Verification items for the finished model (mm, model axes). A direction names the side the tool comes from. Coordinates: 2 decimals unless noted, no trailing zeros. Write each loop counter-clockwise with the first axis right and the second up, starting at its lowest first coordinate (ties: lowest second). Pieces come first, ordered by that corner, then holes. Notation, with made-up numbers: (60.5, -5) -> (80.5, -5) arc R21 ccw to (80.5, 24) -> close; hole circle Ø2 at (-11.5, 78.5). An arc over 180 degrees is marked (long way). Use a Markdown table: item, result. Add a question column.
from build123d import *

# Parameters (mm, degrees)
EXTRUSION1_DEPTH        = 5.25
CONG_1_R                = 2
ENL_V_MAT_EXTRU_1_DEPTH = 2.5


with BuildPart() as part:
    # Esquisse1 → Extrusion1 (new body, symmetric)
    with BuildSketch(Plane.XY):
        with BuildLine():
            Line((4.5, 8), (-4.5, 8))
            Line((-4.5, 8), (-9.009706909, 21.487495824))
            ThreePointArc((-9.009706909, 21.487495824), (0, 34), (9.009706909, 21.487495824))
            Line((9.009706909, 21.487495824), (4.5, 8))
        make_face()
    extrude(amount=EXTRUSION1_DEPTH, both=True)

    # Congé1
    cong_1_edges = [part.edges().sort_by_distance(p)[0] for p in [
        (6.754853455, 14.743747912, 5.25),
        (0, 34, 5.25),
        (-6.754853455, 14.743747912, 5.25),
        (0, 34, -5.25),
        (6.754853455, 14.743747912, -5.25),
        (-6.754853455, 14.743747912, -5.25),
    ]]
    fillet(cong_1_edges, radius=CONG_1_R)

    # Esquisse3 → Révolution2 (revolve)
    with BuildSketch(Plane.XY, mode=Mode.PRIVATE) as r_volution2_sk:
        Polygon((-13.067694578, 46.211312018), (-9.438866144, 31.656876124), (-7.983422555, 32.019758967), (-6.345144878, 25.448986095), (-9.498605988, 24.662739935), (-14.037990304, 45.969390122), align=None)
    r_volution2 = revolve(r_volution2_sk.sketch.rotate(Axis((0, 0, 0), (-0.241921896, 0.970295726, 0)), 180), axis=Axis((0, 0, 0), (-0.241921896, 0.970295726, 0)))  # turned: the seam where the file's is

    # Symétrie1: Révolution2 across plane
    add(r_volution2.mirror(Plane(origin=(0, 0, 0), x_dir=(0, 0, 1), z_dir=(1, 0, 0))))

    # Esquisse5 → Enlèv. mat.-Extru.1 (cut, symmetric)
    with BuildSketch(Plane(origin=(0, 0, 0), x_dir=(0, 0, -1), z_dir=(1, 0, 0))):
        with BuildLine():
            Line((-3.25, 8), (3.25, 8))
            Line((3.25, 8), (3.25, 10))
            Line((3.25, 10), (2.291287847, 10))
            ThreePointArc((2.291287847, 10), (0, 13.5), (-2.291287847, 10))
            Line((-2.291287847, 10), (-3.25, 10))
            Line((-3.25, 10), (-3.25, 8))
        make_face()
    extrude(amount=ENL_V_MAT_EXTRU_1_DEPTH, both=True, mode=Mode.SUBTRACT)


solid = part.part
1) Cross-section at A-A on x = 0. Record the boundary of the cut face in (y, z), then the cut area to 3 significant figures.
2) Thickness scan on L1, parallel to Z at x = 1, y = 11; L2, parallel to X at y = 23.5, z = -3; L3, parallel to X at y = 36.5, z = 2. Record the ranges inside material, lowest first.
3) Cross-section at B-B on z = 4. Record the boundary of the cut face in (x, y).
4) Gauge pin test, flat ends, axial feed: pin 1 (1.1 mm diameter, centred on x = 0, z = -3, fed in from -Y); pin 2 (5 mm diameter, centred on y = 39, z = 3.5, fed in from -X); pin 3 (3 mm diameter, centred on y = 35, z = -3.5, fed in from -X); pin 4 (6 mm diameter, centred on x = 0.5, y = 39.5, fed in from +Z). Record the tip position at first contact, or that the pin passes through.
5) Cross-section at C-C on y = 37.5. Give the number of separate pieces and of enclosed holes in the cut face, then the cut area to 3 significant figures.
6) Release check for a two-part mould opening along Y. For faces 1 (the face through (8.004, 32.015, -0.021)), 2 (the face through (-10.03, 46.97, 0.52)), 3 (the face through (-3, 8, 0)) record: released by +Y, released by -Y, zero draft, split by the parting line, or undercut.
7) Set-up check for faces 4 (the face through (0, 10, 3)), 5 (the face through (0, 13.5, -0.1)), 6 (the face through (-6.11, 14.72, 4.68)): record each of +Z, -Z, +X, -X, +Y, -Y from which the full face is reachable in a straight line by a thin tool's end or side.
Returned:
| question | item | result |
|---|---|---|
| 1 | outline | (8, -5.25) -> (32, -5.25) arc R2 ccw to (34, -3.25) -> (34, 3.25) arc R2 ccw to (32, 5.25) -> (8, 5.25) -> (8, 3.25) -> (10, 3.25) -> (10, 2.29) arc R2.5 cw (long way) to (10, -2.29) -> (10, -3.25) -> (8, -3.25) -> close |
| 1 | area | 244 mm² |
| 2 | L1 | z = -5.25 to -2.5, 2.5 to 5.25 |
| 2 | L2 | x = -9.45 to 9.45 |
| 2 | L3 | x = -11.18 to -6.97, 6.97 to 11.18 |
| 3 | outline | (-8.87, 21.53) -> (-4.35, 8) -> (4.35, 8) -> (8.87, 21.53) arc R9.35 ccw (long way) to start |
| 4 | pin 1 | stops at y = 8 |
| 4 | pin 2 | stops at x = -12.48 |
| 4 | pin 3 | stops at x = -10.91 |
| 4 | pin 4 | passes through |
| 5 | separate pieces | 2 |
| 5 | enclosed holes | 2 |
| 5 | area | 37.0 mm² |
| 6 | face 1 | undercut |
| 6 | face 2 | released by +Y |
| 6 | face 3 | released by -Y |
| 7 | face 4 | -Y |
| 7 | face 5 | none |
| 7 | face 6 | +Z, -X, -Y |
